Build history of the part. All positions in model axes, mm. Face numbers are marked on the shaded views. A direction names the side the tool comes from. Round coordinates to 2 decimals unless told otherwise and drop trailing zeros. Write each loop counter-clockwise with the first axis right and the second up, starting at its lowest first coordinate (ties: lowest second). Pieces come first, ordered by that corner, then holes.
1) Pull direction X, two halves, no side cores. Call the marked faces 3, 4 and 5: +X half, -X half, draft (parallel to the pull), parting line (faces both ways), or undercut.
2) Saw through at C-C (y = 4). Write the cut outline in (x, z) (3 decimals), plus the area to 3 significant figures.
3) Wall check: probe 1 along X at (y, z) = (6.25, -19.5) (3 decimals); probe 2 along Y at (x, z) = (2, -32.5) (3 decimals); probe 3 along Z at (x, y) = (2.25, 1.75). Give the ranges that are in metal, low to high.
4) Which spindle directions (+Z, -Z, +X, -X, +Y, -Y) get a long thin tool onto all of the face, cutting with end or side? Do the marked faces 1 and 2. Say none if no direction does.
5) Saw through at D-D (y = 0.75). Write the cut outline in (x, z) (3 decimals), plus the area to 3 significant figures.
6) Saw through at A-A (x = 2.54). Write the cut outline in (y, z) (3 decimals), plus the area to 3 significant figures.
7) Flat gauge pins, fed straight in: pin 1 (2 mm diameter, centred on y = 3, z = -40.5, fed in from -X); pin 2 (3 mm diameter, centred on x = 2, z = -5.5, fed in from +Y) (3 decimals); pin 3 (3.5 mm diameter, centred on x = 2.54, z = -44.45, fed in from -Y); pin 4 (1 mm diameter, centred on x = -2.5, y = 1, fed in from -Z). Where does each tip first touch, or does it go through?
8) Saw through at B-B (z = 6.35). Write the cut outline in (x, y).
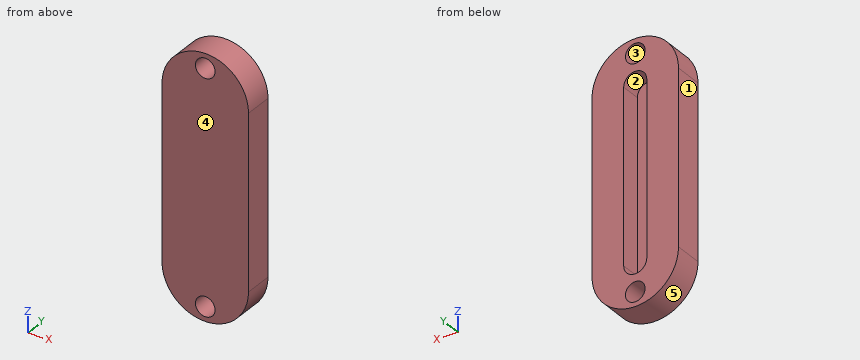
from build123d import *

# Parameters (mm, degrees)
BOSS_EXTRUDE1_DEPTH = 6.35
BOSS_EXTRUDE2_DEPTH = 1.905
SKETCH3_R           = 2.159
CUT_EXTRUDE1_DEPTH  = 12.7


with BuildPart() as part:
    # Sketch1 → Boss-Extrude1 (new body)
    with BuildSketch(Plane(origin=(0, 0, 0), x_dir=(1, 0, 0), z_dir=(0, 1, 0))):
        with BuildLine():
            Line((-6.985, 38.1), (-6.985, 0))
            ThreePointArc((-6.985, 0), (2.54, -9.525), (12.065, 0))
            Line((12.065, 0), (12.065, 38.1))
            ThreePointArc((12.065, 38.1), (2.54, 47.625), (-6.985, 38.1))
        make_face()
        with BuildLine():
            Line((0, 0), (0, 38.1))
            ThreePointArc((0, 38.1), (2.54, 40.64), (5.08, 38.1))
            Line((5.08, 38.1), (5.08, 0))
            ThreePointArc((5.08, 0), (2.54, -2.54), (0, 0))
        make_face(mode=Mode.SUBTRACT)
    extrude(amount=BOSS_EXTRUDE1_DEPTH)

    # Sketch2 → Boss-Extrude2 (add)
    with BuildSketch(Plane(origin=(0, 0, 0), x_dir=(1, 0, 0), z_dir=(0, 1, 0))):
        with BuildLine():
            Line((0, 38.1), (0, 0))
            ThreePointArc((0, 0), (2.54, -2.54), (5.08, 0))
            Line((5.08, 0), (5.08, 38.1))
            ThreePointArc((5.08, 38.1), (2.54, 40.64), (0, 38.1))
        make_face()
    extrude(amount=BOSS_EXTRUDE2_DEPTH)

    # Sketch3 → Cut-Extrude1 (cut)
    with BuildSketch(Plane(origin=(0, 6.35, 0), x_dir=(1, 0, 0), z_dir=(0, 1, 0))):
        with Locations(Location((2.54, 44.45, 0), (0, 0, 270))):
            Circle(SKETCH3_R)
        with Locations(Location((2.54, -6.35, 0), (0, 0, 270))):
            Circle(SKETCH3_R)
    extrude(amount=-CUT_EXTRUDE1_DEPTH, mode=Mode.SUBTRACT)


solid = part.part
Evaluation:
1. face 3: undercut
1. face 4: draft
1. face 5: parting line
2. outline: (-6.985, -38.1) arc R9.525 ccw to (12.065, -38.1) - (12.065, 0) arc R9.525 ccw to (-6.985, 0) - close; hole (0, -38.1) arc R2.54 ccw to (5.08, -38.1) - (5.08, 0) arc R2.54 ccw to (0, 0) - close; hole circle Ø4.318 at (2.54, -44.45); hole circle Ø4.318 at (2.54, 6.35)
2. area: 768 mm2
3. probe 1: x = -6.985 to 0, 5.08 to 12.065
3. probe 2: y = 0 to 1.905
3. probe 3: z = -47.62 to -46.59, -42.31 to 4.21, 8.49 to 9.52
4. face 1: +Z, -Z, -X, +Y, -Y
4. face 2: +Y
5. outline: (-6.985, -38.1) arc R9.525 ccw to (12.065, -38.1) - (12.065, 0) arc R9.525 ccw to (-6.985, 0) - close; hole circle Ø4.318 at (2.54, -44.45); hole circle Ø4.318 at (2.54, 6.35)
5. area: 982 mm2
6. outline: (0, -47.625) - (6.35, -47.625) - (6.35, -46.609) - (0, -46.609) - close; (0, -42.291) - (6.35, -42.291) - (6.35, -40.64) - (1.905, -40.64) - (1.905, 2.54) - (6.35, 2.54) - (6.35, 4.191) - (0, 4.191) - close; (0, 8.509) - (6.35, 8.509) - (6.35, 9.525) - (0, 9.525) - close
6. area: 116 mm2
7. pin 1: stops at x = -6.88
7. pin 2: stops at y = 1.905
7. pin 3: passes through
7. pin 4: stops at z = -46.47
8. outline: (-4.56, 0) - (0.38, 0) - (0.38, 6.35) - (-4.56, 6.35) - close; (4.7, 0) - (9.64, 0) - (9.64, 6.35) - (4.7, 6.35) - close
